```python
from build123d import *

# Parameters (mm, degrees)
F0_W      = 8.3522722125
F0_H      = 65.1477314532
F1_DEPTH  = 19.841
F2_W      = 8.3522722125
F2_H      = 11.6972830147
F3_DEPTH  = 15
F3_FACE_W = 8.3522722125
F3_FACE_H = 11.6972830147
F1_FACE_W = 8.3522722125
F1_FACE_H = 53.4504484385
F5_DEPTH  = 65


with BuildPart() as f1:
    # F0 (on Top) → F1 (new body)
    with BuildSketch(Plane.XY):
        with Locations((9.7681805491, -0.9545441717)):
            Rectangle(F0_W, F0_H)
    extrude(amount=F1_DEPTH)

    # F2 (on face) → F3 (join)
    with BuildSketch(Plane.XY.offset(19.841)):
        with Locations((9.7681805491, -27.679768391)):
            Rectangle(F2_W, F2_H)
    extrude(amount=F3_DEPTH)

    # F3_face (on face) → F4 section 0
    with BuildSketch(Plane(origin=(9.7681805491, -27.679768391, 34.841), x_dir=(1, 0, 0), z_dir=(0, 0, 1))):
        Rectangle(F3_FACE_W, F3_FACE_H)
    # F1_face (on face) → F4 section 1
    with BuildSketch(Plane(origin=(9.7681805491, -0.9545441717, 19.841), x_dir=(1, 0, 0), z_dir=(0, 0, 1))):
        with Locations((0, 5.8486415073)):
            Rectangle(F1_FACE_W, F1_FACE_H)
    loft(mode=Mode.SUBTRACT)

    # F5 (add): a face of the model
    f5_faces = [f1.faces().sort_by_distance(p)[0] for p in [
        (9.7681805491, 31.6193215549, 9.9205),
    ]]
    extrude(f5_faces, amount=F5_DEPTH)


solid = f1.part
```
Verification items for the finished model (mm, model axes). A direction names the side the tool comes from. Round coordinates to 2 decimals unless told otherwise and drop trailing zeros. Write each loop counter-clockwise with the first axis right and the second up, starting at its lowest first coordinate (ties: lowest second). Pieces come first, ordered by that corner, then holes.
1. Scan lines: L1, parallel to Z at x = 13.25, y = -15; L2, parallel to Y at x = 8.25, z = 27.5; L3, parallel to Y at x = 13.25, z = 21. Record each from-to range of solid material in increasing order.
2. Section check C-C on z = 26. Enter the section's corners in (x, y).
3. Section check B-B on y = 16. Enter the section's corners in (x, z).
4. Section check A-A on x = 8. Enter the section's corners in (y, z).
5. Access from +Z, -Z, +X, -X, +Y, -Y to the whole of each face (thin tool, end or side, straight path). Record for faces 1 (the flat face through (10, 37, 19.841)), 2 (the flat face through (5.592, 31, 9)).
Answer:
1. L1: z = 0 to 19.84
1. L2: y = -33.53 to -27.8
1. L3: y = -33.53 to -22.73
2. outline: (5.59, -33.53) - (13.94, -33.53) - (13.94, -26.63) - (5.59, -26.63) - close
3. outline: (5.59, 0) - (13.94, 0) - (13.94, 19.84) - (5.59, 19.84) - close
4. outline: (-33.53, 0) - (96.62, 0) - (96.62, 19.84) - (-21.83, 19.84) - (-33.53, 34.84) - close
5. face 1: +Z, +X, -X, +Y
5. face 2: +Z, -Z, -X, +Y, -Y
